Build history of the part. All positions in model axes, mm. A direction names the side the tool comes from. Give positions to 0.01 mm unless a question says otherwise; leave off trailing zeros. Loops run counter-clockwise (first coordinate to the right, second up) from the corner with the lowest first, then second, coordinate; pieces in that order, holes last. Notation, with made-up numbers: M 23.25,64.25 L 62.25,64.25 A22 ccw 62.25,92.25 Z; hole C 41,41 d10. An arc over 180 degrees is marked long. Put each result on its own line as item: value.
```python
from build123d import *

# Parameters (mm, degrees)
SKETCH7_R               = 2.75
BOSS_EXTRUDE5_DEPTH     = 5
FILLET4_R               = 10
SKETCH8_R               = 2.75
BOSS_EXTRUDE6_DEPTH     = 5
SKETCH9_W               = 10
SKETCH9_H               = 10
SKETCH9_H_2             = 40
SKETCH9_W_2             = 5
BOSS_EXTRUDE7_DEPTH     = 7.5
FILLET5_R               = 5
SKETCH10_R              = 2.75
CUT_EXTRUDE3_DEPTH      = 64.495460213
SKETCH11_R              = 2.75
BOSS_EXTRUDE8_DEPTH     = 5
BOSS_EXTRUDE9_DEPTH     = 5
FILLET6_R               = 5
CUT_EXTRUDE4_START      = -5
SKETCH13_R              = 2.75
CUT_EXTRUDE4_DEPTH      = 5
CUT_EXTRUDE5_DEPTH      = 127.477470595
CUT_EXTRUDE5_DEPTH_BACK = 127.477470595
SKETCH14_R              = 2.75


with BuildPart() as part:
    # Sketch7 → Boss-Extrude5 (new body)
    with BuildSketch(Plane.XY):
        with BuildLine():
            Line((72.320508076, 39.737205584), (55, 29.737205584))
            ThreePointArc((55, 29.737205584), (51.339745962, 16.076951546), (65, 12.416697508))
            ThreePointArc((65, 12.416697508), (61.339745962, -1.24355653), (75, -4.903810568))
            Line((75, -4.903810568), (92.320508076, 5.096189432))
            Line((92.320508076, 5.096189432), (72.320508076, 39.737205584))
        make_face()
        with Locations((70, 3.75644347)):
            Circle(SKETCH7_R, mode=Mode.SUBTRACT)
        with Locations((60, 21.076951546)):
            Circle(SKETCH7_R, mode=Mode.SUBTRACT)
    extrude(amount=BOSS_EXTRUDE5_DEPTH)

    # Fillet4
    fillet4_edges = [part.edges().sort_by_distance(p)[0] for p in [
        (65, 12.416697508, 2.5),
    ]]
    fillet(fillet4_edges, radius=FILLET4_R)



with BuildPart() as body_2:
    # Sketch8 → Boss-Extrude6 (new body)
    with BuildSketch(Plane(origin=(0, 0, -10), x_dir=(-1, 0, 0), z_dir=(0, 0, -1))):
        with BuildLine():
            Line((-55, 29.737205584), (-72.320508076, 39.737205584))
            Line((-72.320508076, 39.737205584), (-92.320508076, 5.096189432))
            Line((-92.320508076, 5.096189432), (-75, -4.903810568))
            ThreePointArc((-75, -4.903810568), (-65, -4.903810568), (-60, 3.75644347))
            ThreePointArc((-60, 3.75644347), (-58.660254038, 8.75644347), (-55, 12.416697508))
            ThreePointArc((-55, 12.416697508), (-50, 21.076951546), (-55, 29.737205584))
        make_face()
        with Locations(Location((-70, 3.75644347, 0), (0, 0, 180))):
            Circle(SKETCH8_R, mode=Mode.SUBTRACT)
        with Locations(Location((-60, 21.076951546, 0), (0, 0, 180))):
            Circle(SKETCH8_R, mode=Mode.SUBTRACT)
    extrude(amount=BOSS_EXTRUDE6_DEPTH)


with BuildPart() as part_1:
    add(part.part)

    add(body_2.part)  # Boss-Extrude7 merges body 2
    # Sketch9 → Boss-Extrude7 (add)
    with BuildSketch(Plane(origin=(71.447095812, 41.25, 0), x_dir=(0, 0, -1), z_dir=(0.8660254037844416, 0.4999999999999949, 0))):
        with Locations((5, 3.253175473)):
            Rectangle(SKETCH9_W, SKETCH9_H)
        Polygon((0, 8.253175473), (-15, 8.253175473), (-15, -51.746824527), (25, -51.746824527), (25, 8.253175473), (10, 8.253175473), (10, -1.746824527), (15, -1.746824527), (15, -41.746824527), (10, -41.746824527), (0, -41.746824527), (-5, -41.746824527), (-5, -1.746824527), (0, -1.746824527), align=None)
        with Locations((5, -21.746824527)):
            Rectangle(SKETCH9_W, SKETCH9_H_2)
        with Locations((12.5, -21.746824527)):
            Rectangle(SKETCH9_W_2, SKETCH9_H_2)
        with Locations((-2.5, -21.746824527)):
            Rectangle(SKETCH9_W_2, SKETCH9_H_2)
    extrude(amount=BOSS_EXTRUDE7_DEPTH)

    # Fillet5
    fillet5_edges = [part_1.edges().sort_by_distance(p)[0] for p in [
        (70.56810334, 50.272459622, -25),
        (70.56810334, 50.272459622, 15),
        (100.56810334, -1.689064606, 15),
        (100.56810334, -1.689064606, -25),
    ]]
    fillet(fillet5_edges, radius=FILLET5_R)

    # Sketch10 → Cut-Extrude3 (cut, through all)
    with BuildSketch(Plane(origin=(77.942286341, 45, 0), x_dir=(0, 0, -1), z_dir=(0.8660254037844415, 0.4999999999999951, 0))):
        with Locations(Location((-9.292893219, 2.546068692, 0), (0, 0, 90))):
            Circle(SKETCH10_R)
        with Locations(Location((19.292893219, 2.546068692, 0), (0, 0, 90))):
            Circle(SKETCH10_R)
        with Locations(Location((19.292893219, -46.039717746, 0), (0, 0, 90))):
            Circle(SKETCH10_R)
        with Locations(Location((-9.292893219, -46.039717746, 0), (0, 0, 90))):
            Circle(SKETCH10_R)
    extrude(amount=-CUT_EXTRUDE3_DEPTH, mode=Mode.SUBTRACT)

    # Sketch11 → Boss-Extrude8 (add)
    with BuildSketch(Plane.XY):
        with BuildLine():
            Line((48.660254038, 60.717967697), (68.660254038, 26.076951546))
            ThreePointArc((68.660254038, 26.076951546), (65, 12.416697508), (51.339745962, 16.076951546))
            Line((51.339745962, 16.076951546), (31.339745962, 50.717967697))
            ThreePointArc((31.339745962, 50.717967697), (35, 64.378221735), (48.660254038, 60.717967697))
        make_face()
        with Locations((40, 55.717967697)):
            Circle(SKETCH11_R, mode=Mode.SUBTRACT)
        with Locations((60, 21.076951546)):
            Circle(SKETCH11_R, mode=Mode.SUBTRACT)
    extrude(amount=BOSS_EXTRUDE8_DEPTH)

    # Sketch12 → Boss-Extrude9 (add)
    with BuildSketch(Plane(origin=(0, 0, -10), x_dir=(-1, 0, 0), z_dir=(0, 0, -1))):
        with BuildLine():
            Line((-48.660254038, 60.717967697), (-63.660254038, 34.737205584))
            Line((-63.660254038, 34.737205584), (-72.320508076, 39.737205584))
            Line((-72.320508076, 39.737205584), (-92.320508076, 5.096189432))
            Line((-92.320508076, 5.096189432), (-75, -4.903810568))
            ThreePointArc((-75, -4.903810568), (-65, -4.903810568), (-60, 3.75644347))
            ThreePointArc((-60, 3.75644347), (-58.660254038, 8.75644347), (-55, 12.416697508))
            ThreePointArc((-55, 12.416697508), (-52.928932188, 14.005883734), (-51.339745962, 16.076951546))
            Line((-51.339745962, 16.076951546), (-31.339745962, 50.717967697))
            ThreePointArc((-31.339745962, 50.717967697), (-35, 64.378221735), (-48.660254038, 60.717967697))
        make_face()
    extrude(amount=BOSS_EXTRUDE9_DEPTH)

    # Fillet6
    fillet6_edges = [part_1.edges().sort_by_distance(p)[0] for p in [
        (92.320508076, 5.096189432, -12.5),
        (92.320508076, 5.096189432, 2.5),
        (72.320508076, 39.737205584, -12.5),
        (72.320508076, 39.737205584, 2.5),
        (63.660254038, 34.737205584, -12.5),
        (63.660254038, 34.737205584, 2.5),
    ]]
    fillet(fillet6_edges, radius=FILLET6_R - 0.0001)  # a hair under: the kernel refuses the full size

    # Sketch13 → Cut-Extrude4 (cut)
    with BuildSketch(Plane.XY.offset(-10).offset(CUT_EXTRUDE4_START)):
        with Locations((40, 55.717967697)):
            Circle(SKETCH13_R)
    extrude(amount=CUT_EXTRUDE4_DEPTH, mode=Mode.SUBTRACT)

    # Sketch14 → Cut-Extrude5 (cut, two sides: drawn at the far end of the back side and taken through both)
    with BuildSketch(Plane.XY.offset(5).offset(-CUT_EXTRUDE5_DEPTH_BACK)):
        with Locations((60, 21.076951546)):
            Circle(SKETCH14_R)
        with Locations((70, 3.75644347)):
            Circle(SKETCH14_R)
    extrude(amount=CUT_EXTRUDE5_DEPTH + CUT_EXTRUDE5_DEPTH_BACK, mode=Mode.SUBTRACT)


solid = part_1.part
```
Q1. Mould opens along Y. For faces 1 (the flat face through (41.48, 33.155, 2.465)), 2 (the flat face through (88.606, 26.53, -4.72)), 3 (the cylindrical face through (74.841, 42.977, 9.414)) say: pulls with the +Y half, pulls with the -Y half, needs draft (parallel to the pull), parting line crosses it, or undercut.
Here are the results:
face 1: pulls with the -Y half
face 2: pulls with the +Y half
face 3: undercut
Q2. Slice it at C-C (z = 2). State how many separate pieces and enclosed holes the cut face has, and give its area (3 significant figures).
Here are the results:
separate pieces: 1
enclosed holes: 3
area: 2,300 mm²
Q3. Probe line 1 (Z direction, x = 73, y = 16); line 2 (Y direction, x = 70, z = -11.15); line 3 (Y direction, x = 40.5, z = 3.5). List the from-to ranges inside material, lowest first. Write a range as from..to.
Here are the results:
line 1: -15..-10, 0..5
line 2: -6.24..1.01, 6.51..39.41, 43.73..49.94
line 3: 34.85..53.01, 58.42..65.71
Q4. Drop flat-ended pins along their axis: pin 1 Ø7 at (x, y) = (40, 55.72) entering from +Z; pin 2 Ø6 at (y, z) = (23, 4) entering from +X; pin 3 Ø19.5 at (x, y) = (56, 44) entering from -Z; pin 4 Ø10 at (x, y) = (95.5, 21.5) entering from -Z. Give the stop position or say it passes through.
Here are the results:
pin 1: z = 5
pin 2: x = 92.38
pin 3: z = -15
pin 4: z = -25
Q5. Slice it at A-A (x = 40). List the corners of the cut face in (y, z), and give its area (3 significant figures).
Here are the results:
outline: M 35.72,-15 L 52.97,-15 L 52.97,-10 L 35.72,-10 Z; M 35.72,0 L 52.97,0 L 52.97,5 L 35.72,5 Z; M 58.47,-15 L 65.72,-15 L 65.72,-10 L 58.47,-10 Z; M 58.47,0 L 65.72,0 L 65.72,5 L 58.47,5 Z
area: 245 mm²
Q6. Slice it at B-B (x = 83). List the corners of the cut face in (y, z) (3 decimals).
Here are the results:
outline: M -0.285,-15 L 21.24,-15 L 21.24,-25 L 36.24,-25 L 36.24,15 L 21.24,15 L 21.24,5 L -0.285,5 L -0.285,0 L 21.24,0 L 21.24,-10 L -0.285,-10 Z
Q7. Tool access for faces 4 (the flat face through (81.4, -1.21, 2.46)), 5 (the cylindrical face through (52.903, 14.032, 2.465)), 6 (the flat face through (70.523, 50.246, -5.21)): list every direction of +Z, -Z, +X, -X, +Y, -Y with a clear straight run to the whole face (end or side of a thin tool).
Here are the results:
face 4: +Z, -Z, -Y
face 5: +Z, -Z, -X, -Y
face 6: +Z, -Z, +Y
